Job drawing, mm, ordinate dimensions from the low corner. One solid piece. A direction names the side the tool comes from. Give positions to 0.01 mm unless a question says otherwise; leave off trailing zeros. Loops run counter-clockwise (first coordinate to the right, second up) from the corner with the lowest first, then second, coordinate; pieces in that order, holes last.
Item 1: Saw through at A-A on z = 6. Give the cut face in (x, y), plus the area to 3 significant figures.
Item 2: Saw through at D-D on z = 16.25. Give the cut face in (x, y).
Item 3: Which spindle directions (+Z, -Z, +X, -X, +Y, -Y) get a long thin tool onto all of the face, cutting with end or side? Do the marked faces 1, 2, 3 and 4. Say none if no direction does.
Item 4: Saw through at C-C on y = 18. Give the cut face in (x, z).
Item 5: Mould opens along Y. For the marked faces 5, 6 and 7 say: released by +Y, released by -Y, zero draft, split by the parting line, or undercut.
Item 6: Drop flat-ended pins along their axis: P1, Ø3, axis at y = 21, z = 5.5, coming from the -X side; P2, Ø4, axis at x = 111, z = 7, coming from the +Y side; P3, Ø4, axis at x = 52.5, z = 5, coming from the -Y side. Give the stop position or say it passes through.
Item 7: Saw through at B-B on x = 130.5. Give the cut face in (y, z).
Item 8: Probe probe 1 along Y at (x, z) = (17, 16.75); probe 2 along X at (y, z) = (12, 10.75); probe 3 along X at (y, z) = (16, 22.25). List the from-to ranges inside material, lowest first.
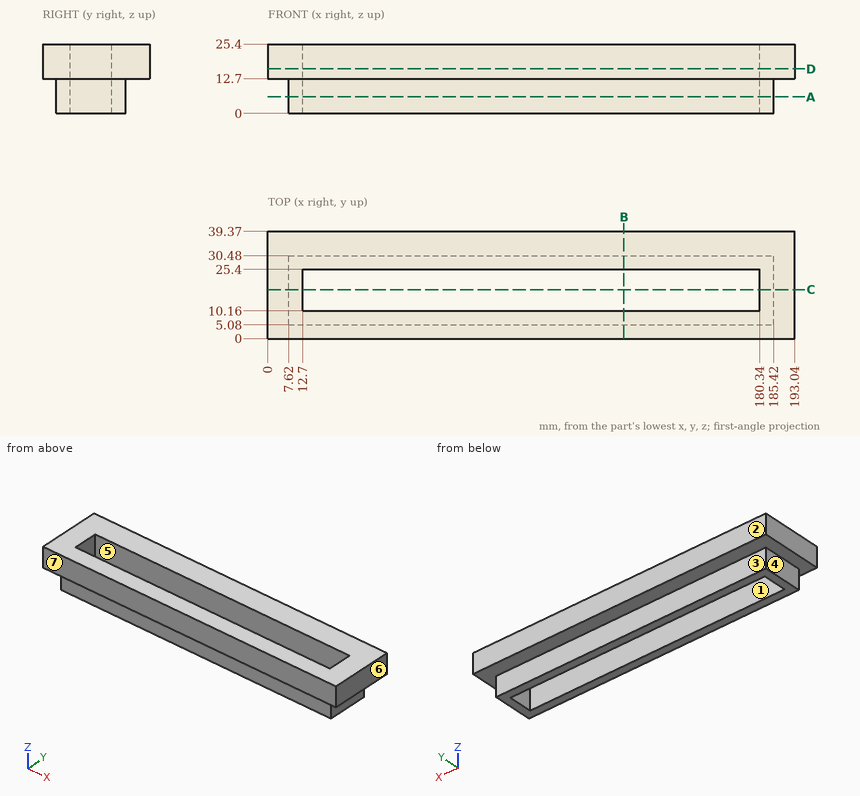
Results below:
1. outline: (7.62, 5.08) - (185.42, 5.08) - (185.42, 30.48) - (7.62, 30.48) - close; hole (12.7, 10.16) - (180.34, 10.16) - (180.34, 25.4) - (12.7, 25.4) - close
1. area: 1,960 mm2
2. outline: (0, 0) - (193.04, 0) - (193.04, 39.37) - (0, 39.37) - close; hole (12.7, 10.16) - (180.34, 10.16) - (180.34, 25.4) - (12.7, 25.4) - close
3. face 1: +Z, -Z
3. face 2: +Z, -Z, +X, -X, +Y
3. face 3: -Z, +X, -X, +Y
3. face 4: -Z, -X, +Y, -Y
4. outline: (0, 12.7) - (7.62, 12.7) - (7.62, 0) - (12.7, 0) - (12.7, 25.4) - (0, 25.4) - close; (180.34, 0) - (185.42, 0) - (185.42, 12.7) - (193.04, 12.7) - (193.04, 25.4) - (180.34, 25.4) - close
5. face 5: undercut
5. face 6: zero draft
5. face 7: released by -Y
6. P1: stops at x = 7.62
6. P2: stops at y = 30.48
6. P3: stops at y = 5.08
7. outline: (0, 12.7) - (5.08, 12.7) - (5.08, 0) - (10.16, 0) - (10.16, 25.4) - (0, 25.4) - close; (25.4, 0) - (30.48, 0) - (30.48, 12.7) - (39.37, 12.7) - (39.37, 25.4) - (25.4, 25.4) - close
8. probe 1: y = 0 to 10.16, 25.4 to 39.37
8. probe 2: x = 7.62 to 12.7, 180.34 to 185.42
8. probe 3: x = 0 to 12.7, 180.34 to 193.04
